Source: CAD feature listing. Evaluate the final solid. Frame: model axes, mm. Round coordinates to 2 decimals unless told otherwise and drop trailing zeros. Order: outer loops, then holes, each group sorted by start corner. A loop starts at its lowest first (then second) coordinate and runs counter-clockwise, first axis right, second up. Notation, with made-up numbers: (25.5, 26) -> (69.5, 26) arc R29 cw to (69.5, 54) -> close; hole circle Ø10 at (27, -6). An arc over 180 degrees is marked (long way). Answer as CSV lines item,"result". Start each with the question number.
(1) Contact query for a flat-ended pin moving along its axis: P1, Ø3.5, axis at x = -21.5, y = -22.5, coming from the +Z side. Output: stop coordinate, or through.
(2) Pull-direction query (X, two-part tool) for faces 1 (the cylindrical face through (24.247, -22.379, 2.465)), 2 (the flat face through (41.5, -23, 2)), 3 (the flat face through (-1, -22, 0)); classes: +X half, -X half, draft (parallel to the pull), parting line (faces both ways), or undercut.
(3) Section query D-D (x = 34). Output: boundary loops of the cut face in (y, z), plus the area to 3 significant figures.
(4) Section query C-C (x = 21.5). Output: boundary loops of the cut face in (y, z), plus the area to 3 significant figures.
(5) Section query B-B (z = 2.6). Output: boundary loops of the cut face in (x, y).
(6) Section query A-A (y = -22.5). Output: boundary loops of the cut face in (x, z).
(7) Line query: line 1 along Y through (x, z) = (21.5, 3.2); line 2 along X through (y, z) = (-24.5, 3.85); line 3 along X through (y, z) = (-21, 2.85). Output: solid intervals per line, ascending. Write a range as from..to.
```python
from build123d import *

# Parameters (mm, degrees)
SKETCH1_W            = 83
SKETCH1_H            = 67
BOSS_EXTRUDE1_DEPTH  = 5
M5_CLEARANCE_HOLE1_D = 5.5
M3_CLEARANCE_HOLE1_D = 3.4
SKETCH6_R            = 11.05
CUT_EXTRUDE1_DEPTH   = 6
FILLET1_R            = 10
SKETCH7_W            = 96.913580025
SKETCH7_H            = 48.46217056
CUT_EXTRUDE2_DEPTH   = 6
FILLET2_R            = 10


with BuildPart() as part:
    # Sketch1 → Boss-Extrude1 (new body)
    with BuildSketch(Plane.XY):
        Rectangle(SKETCH1_W, SKETCH1_H)
    extrude(amount=BOSS_EXTRUDE1_DEPTH)

    # M5 Clearance Hole1 (through all)
    with Locations(Plane.XY.offset(5)):
        with Locations((21.5, -22.5), (-21.5, -22.5)):
            Hole(M5_CLEARANCE_HOLE1_D / 2)

    # M3 Clearance Hole1 (through all)
    with Locations(Plane(origin=(0, 0, 0), x_dir=(-1, 0, 0), z_dir=(0, 0, -1))):
        with Locations((-32.041076253, 28.00000478), (-1.041076253, 28.00000478), (-1.041076253, -2.99999522), (-32.041076253, -2.99999522)):
            Hole(M3_CLEARANCE_HOLE1_D / 2)

    # Sketch6 → Cut-Extrude1 (cut, through all)
    with BuildSketch(Plane.XY.offset(5)):
        with Locations((16.541076624, 12.500005008)):
            Circle(SKETCH6_R)
    extrude(amount=-CUT_EXTRUDE1_DEPTH, mode=Mode.SUBTRACT)

    # Fillet1
    fillet1_edges = [part.edges().sort_by_distance(p)[0] for p in [
        (41.5, -33.5, 2.5),
        (-41.5, -33.5, 2.5),
        (-41.5, 33.5, 2.5),
        (41.5, 33.5, 2.5),
    ]]
    fillet(fillet1_edges, radius=FILLET1_R)

    # Sketch7 → Cut-Extrude2 (cut, through all)
    with BuildSketch(Plane.XY.offset(5)):
        with Locations((2.882260535, 12.73108528)):
            Rectangle(SKETCH7_W, SKETCH7_H)
    extrude(amount=-CUT_EXTRUDE2_DEPTH, mode=Mode.SUBTRACT)

    # Fillet2
    fillet2_edges = [part.edges().sort_by_distance(p)[0] for p in [
        (41.5, -11.5, 2.5),
        (-41.5, -11.5, 2.5),
    ]]
    fillet(fillet2_edges, radius=FILLET2_R)


solid = part.part
```
Answer block:
1,P1,"through"
2,face 1,"undercut"
2,face 2,"+X half"
2,face 3,"draft"
3,outline,"(-33.18, 0) -> (-11.82, 0) -> (-11.82, 5) -> (-33.18, 5) -> close"
3,area,"107 mm2"
4,outline,"(-33.5, 0) -> (-25.25, 0) -> (-25.25, 5) -> (-33.5, 5) -> close; (-19.75, 0) -> (-11.5, 0) -> (-11.5, 5) -> (-19.75, 5) -> close"
4,area,"82.5 mm2"
5,outline,"(-41.5, -23.5) arc R10 ccw to (-31.5, -33.5) -> (31.5, -33.5) arc R10 ccw to (41.5, -23.5) -> (41.5, -21.5) arc R10 ccw to (31.5, -11.5) -> (-31.5, -11.5) arc R10 ccw to (-41.5, -21.5) -> close; hole circle Ø5.5 at (-21.5, -22.5); hole circle Ø5.5 at (21.5, -22.5)"
6,outline,"(-41.5, 0) -> (-24.25, 0) -> (-24.25, 5) -> (-41.5, 5) -> close; (-18.75, 0) -> (18.75, 0) -> (18.75, 5) -> (-18.75, 5) -> close; (24.25, 0) -> (41.5, 0) -> (41.5, 5) -> (24.25, 5) -> close"
7,line 1,"-33.5..-25.25, -19.75..-11.5"
7,line 2,"-41.45..-23.39, -19.61..19.61, 23.39..41.45"
7,line 3,"-41.49..-23.8, -19.2..19.2, 23.8..41.49"
